from build123d import *

# Parameters (mm, degrees)
F1_DEPTH = 10
F0_W     = 26
F0_H     = 12
F2_DEPTH = 5
F3_D     = 3
F5_DEPTH = 4.9
F6_D     = 3


with BuildPart() as f1:
    # F0 (on Top) → F1 (new body)
    with BuildSketch(Plane.XY):
        Polygon((20.9, 30.9), (20.9, 16.5), (17.9, 16.5), (17.9, 13.2), (19.4, 11.7), (20.9, 11.7), (20.9, 4.9), (14.1, 4.9), (14.1, 6.4), (12.6, 7.9), (9.3, 7.9), (9.3, 4.9), (-5.1, 4.9), (-5.1, -0.1), (20.9, -0.1), (25.9, 4.9), (25.9, 30.9), align=None)
    extrude(amount=F1_DEPTH)

    # F0 (on Top) → F2 (join)
    with BuildSketch(Plane.XY):
        with Locations((7.9, -6.1)):
            Rectangle(F0_W, F0_H)
    extrude(amount=F2_DEPTH)

    # F3 (through all)
    with Locations(Plane(origin=(0, 0, 0), x_dir=(1, 0, 0), z_dir=(0, 0, -1))):
        with Locations((7.8999996185, 8.1)):
            Hole(F3_D / 2)


with BuildPart() as f5:
    # F4 (on Top) → F5 (new body)
    with BuildSketch(Plane.XY):
        with BuildLine():
            ThreePointArc((20.9, -19.2), (18.8497474683, -14.2502525317), (13.9, -12.2))
            Line((13.9, -12.2), (1.9, -12.2))
            ThreePointArc((1.9, -12.2), (-3.0497474683, -14.2502525317), (-5.1, -19.2))
            Line((-5.1, -19.2), (-5.1, -22.2))
            Line((-5.1, -22.2), (20.9, -22.2))
            Line((20.9, -22.2), (20.9, -19.2))
        make_face()
    extrude(amount=F5_DEPTH)

    # F6 (through all)
    with Locations(Plane(origin=(0, 0, 0), x_dir=(1, 0, 0), z_dir=(0, 0, -1))):
        with Locations((7.9, 16.2)):
            Hole(F6_D / 2)


solid = f5.part
Part model, mm, in its own coordinate system. Give positions to 0.01 mm unless a question says otherwise; leave off trailing zeros. Loops run counter-clockwise (first coordinate to the right, second up) from the corner with the lowest first, then second, coordinate; pieces in that order, holes last. Notation, with made-up numbers: (67.5, 19) -> (113.5, 19) arc R32 cw to (113.5, 57) -> close; hole circle Ø7 at (37, -28). An arc over 180 degrees is marked (long way). Write each question's results on one line, items separated by ' | '. Start each with the question number.
Q1. Pull direction X, two halves, no side cores. Call faces 1 (the face through (7.094, -17.465, 2.484)), 2 (the face through (8, -18, 0)), 3 (the face through (-5.1, -21, 2)): +X half, -X half, draft (parallel to the pull), parting line (faces both ways), or undercut.
Q2. Band-saw the part on C-C on y = -16.2. List the corners of the cut face in (x, z).
Q3. Band-saw the part on B-B on x = 7.9. List the corners of the cut face in (y, z).
Q4. Band-saw the part on A-A on z = 4.3. List the corners of the cut face in (x, y).
Q5. Wall check: L1, parallel to Y at x = 7.9, z = 2.3; L2, parallel to X at y = -16, z = 1.3; L3, parallel to X at y = -16.2, z = 1.3. Give the ranges that are in metal, low to high.
Q6. Band-saw the part on D-D on x = -0.75. List the corners of the cut face in (y, z).
Q7. Pin check, flat tip, straight feed: P1, Ø2, axis at y = -16, z = 1.5, coming from the +X side. Stop position of the tip, or through.
Results are:
1) face 1: undercut | face 2: draft | face 3: -X half
2) outline: (-4.42, 0) -> (6.4, 0) -> (6.4, 4.9) -> (-4.42, 4.9) -> close; (9.4, 0) -> (20.22, 0) -> (20.22, 4.9) -> (9.4, 4.9) -> close
3) outline: (-22.2, 0) -> (-17.7, 0) -> (-17.7, 4.9) -> (-22.2, 4.9) -> close; (-14.7, 0) -> (-12.2, 0) -> (-12.2, 4.9) -> (-14.7, 4.9) -> close
4) outline: (-5.1, -22.2) -> (20.9, -22.2) -> (20.9, -19.2) arc R7 ccw to (13.9, -12.2) -> (1.9, -12.2) arc R7 ccw to (-5.1, -19.2) -> close; hole circle Ø3 at (7.9, -16.2)
5) L1: y = -22.2 to -17.7, -14.7 to -12.2 | L2: x = -4.33 to 6.41, 9.39 to 20.13 | L3: x = -4.42 to 6.4, 9.4 to 20.22
6) outline: (-22.2, 0) -> (-12.72, 0) -> (-12.72, 4.9) -> (-22.2, 4.9) -> close
7) P1: stops at x = 20.55
